Autodesk Inventor part; units mm, degrees
ref_plane "YZ Plane" through (0, 0, 0) normal (1, 0, 0) x (0, 1, 0)
ref_plane "XZ Plane" through (0, 0, 0) normal (0, 1, 0) x (-1, 0, 0)
ref_plane "XY Plane" through (0, 0, 0) normal (0, 0, 1) x (1, 0, 0)
sketch "Sketch1" plane through (0, 0, 0) normal (0, 1, 0) x (-1, 0, 0)
  line L0 (0, 0) -> (-19.6, 0)
  line L1 (-19.6, 0) -> (-19.6, -4)
  line L2 (-19.6, -4) -> (0, -4)
  line L3 (0, -4) -> (0, 0)
  dimension "d0" = 4
  dimension "d1" = 19.6
extrude "Extrusion1" add sketch "Sketch1" along normal blind 34
sketch "Sketch2" plane through (0, 0, -4) normal (-1, 0, 0) x (0, 0, 1)
  line L0 (4, 34) -> (0, 34)
  line L1 (0, 34) -> (8, 34)
  line L2 (8, 34) -> (8, 42)
  line L3 (8, 42) -> (0, 42)
  line L4 (0, 42) -> (0, 34)
  line L5 (4, 0) -> (4, 34)
  dimension "d4" = 4
  dimension "d5" = 8
  dimension "d6" = 8
extrude "Extrusion2" add sketch "Sketch2" against normal blind 32
sketch "Sketch3" plane through (32, 0, -4) normal (1, 0, 0) x (0, 0, -1)
  circle A0 centre (-4, 38) radius 2.5
  line L0 (0, 42) -> (-8, 42)
  line L1 (-8, 42) -> (-8, 34)
  line L2 (0, 34) -> (0, 42)
  line L3 (-8, 34) -> (0, 34)
  point P0 (-4, 0)
  dimension "d9" = 4
  dimension "d10" = 4
  dimension "d11" = 4
  dimension "d12" = 4
  dimension "d13" = 5
extrude "Extrusion3" cut sketch "Sketch3" against normal blind 30.8 contours A0
sketch "Sketch4" plane through (0, 0, 0) normal (0, -1, 0) x (1, 0, 0)
  line L0 (18.4, -3.2) -> (15.6, -3.2)
  line L1 (15.6, -3.2) -> (15.6, -1.6)
  line L2 (15.6, -1.6) -> (18.4, -1.6)
  line L3 (18.4, -1.6) -> (18.4, -3.2)
  line L4 (11.2, -3.2) -> (8.4, -3.2)
  line L5 (8.4, -3.2) -> (8.4, -1.6)
  line L6 (8.4, -1.6) -> (11.2, -1.6)
  line L7 (11.2, -1.6) -> (11.2, -3.2)
  line L8 (4, -3.2) -> (1.2, -3.2)
  line L9 (1.2, -3.2) -> (1.2, -1.6)
  line L10 (1.2, -1.6) -> (4, -1.6)
  line L11 (4, -1.6) -> (4, -3.2)
  line L12 (19.6, 0) -> (19.6, -4)
  line L13 (19.6, -4) -> (0, -4)
  line L14 (0, 0) -> (19.6, 0)
  line L15 (0, -4) -> (0, 0)
  dimension "d16" = 2.8
  dimension "d17" = 1.2
  dimension "d18" = 0.8
  dimension "d19" = 1.6
  dimension "d20" = 1.6
  dimension "d21" = 2.8
  dimension "d22" = 2.8
  dimension "d23" = 4.4
  dimension "d24" = 1.2
  dimension "d25" = 4.4
extrude "Extrusion4" cut sketch "Sketch4" against normal blind 38 contours L0 L1 L2 L3 | L4 L5 L6 L7 | L8 L9 L10 L11
sketch "Sketch5" plane through (19.6, 0, -4) normal (0, 0, -1) x (-1, 0, 0)
  line L0 (1.2, 0) -> (1.2, 38)
  line L1 (4, 0) -> (4, 38)
  line L2 (1.2, 27) -> (4, 27)
  line L3 (4, 27) -> (4, 7)
  line L4 (4, 7) -> (1.2, 7)
  line L5 (1.2, 7) -> (1.2, 27)
  line L6 (8.4, 0) -> (8.4, 36.0791)
  line L7 (11.2, 0) -> (11.2, 38)
  line L8 (8.4, 27) -> (11.2, 27)
  line L9 (11.2, 27) -> (11.2, 7)
  line L10 (11.2, 7) -> (8.4, 7)
  line L11 (8.4, 7) -> (8.4, 27)
  line L12 (15.6, 0) -> (15.6, 36.0791)
  line L13 (15.6, 27) -> (18.4, 27)
  line L14 (18.4, 27) -> (18.4, 7)
  line L15 (18.4, 7) -> (15.6, 7)
  line L16 (15.6, 7) -> (15.6, 27)
  line L17 (0, 0) -> (19.6, 0)
  line L18 (0, 34) -> (-12.4, 34)
  line L19 (19.6, 0) -> (19.6, 42)
  point P0 (18.4, 0)
  point P1 (15.6, 7)
  point P2 (8.4, 7)
  point P3 (1.2, 7)
  point P4 (4, 27)
  dimension "d28" = 7
  dimension "d29" = 20
  dimension "d30" = 7
  dimension "d49" = 1.2
extrude "Extrusion5" cut sketch "Sketch5" against normal blind 0.8 contours L12 L13 L14 L15 | L0 L2 L1 L4 | L6 L8 L7 L10
sketch "Sketch6" plane through (19.6, 0, -4) normal (0, 0, -1) x (-1, 0, 0)
  line L0 (5.2, 27) -> (7.2, 27)
  line L1 (7.2, 27) -> (7.2, 7)
  line L2 (7.2, 7) -> (5.2, 7)
  line L3 (5.2, 7) -> (5.2, 27)
  line L4 (12.4, 27) -> (14.4, 27)
  line L5 (14.4, 27) -> (14.4, 7)
  line L6 (14.4, 7) -> (12.4, 7)
  line L7 (12.4, 7) -> (12.4, 27)
  line L8 (4, 27) -> (4, 7)
  line L9 (8.4, 7) -> (8.4, 27)
  line L10 (11.2, 27) -> (11.2, 7)
  line L11 (15.6, 7) -> (15.6, 27)
  line L12 (19.6, 0) -> (19.6, 42)
  line L13 (0, 0) -> (0, 34)
  dimension "d33" = 1.2
  dimension "d34" = 1.2
  dimension "d35" = 1.2
  dimension "d36" = 1.2
  dimension "d37" = 2
  dimension "d38" = 2
  dimension "d39" = 19.6
extrude "Extrusion6" cut sketch "Sketch6" against normal up to surface (4 mm away)
sketch "Sketch7" plane through (0, 0, 0) normal (0, -1, 0) x (1, 0, 0)
  line L0 (19.6, -4) -> (32, -4)
  line L1 (0, 0) -> (19.6, 0)
  line L2 (19.6, -4) -> (0, -4)
  line L3 (0, -4) -> (0, 0)
  line L4 (0, 0) -> (19.6, 0)
  line L5 (19.6, 0) -> (19.6, -4)
extrude "Extrusion7" add sketch "Sketch7" against normal blind 7
properties part number "20210811_H2_gasmanifold_old_v1"
The listing builds one solid part. Answer for the finished solid, in the listing's coordinates (mm). A direction names the side the tool comes from. Give positions to 0.01 mm unless a question says otherwise; leave off trailing zeros. Order: outer loops, then holes, each group sorted by start corner. A loop starts at its lowest first (then second) coordinate and runs counter-clockwise, first axis right, second up. Notation, with made-up numbers: (24.5, -23) -> (33.5, -23) arc R21 cw to (33.5, -15) -> close; hole circle Ø5 at (62, 77). An arc over 180 degrees is marked (long way). Put each result on its own line as item: value.
Item 1: A cutting plane is placed at C-C on z = 1.5. Give the vertices of the cut face in (x, y), plus the area to 3 significant figures.
Established:
outline: (0, 34) -> (32, 34) -> (32, 36) -> (1.2, 36) -> (1.2, 40) -> (32, 40) -> (32, 42) -> (0, 42) -> close
area: 133 mm^2
Item 2: A cutting plane is placed at D-D on x = 3.5. Give the vertices of the cut face in (y, z).
Established:
outline: (0, -4) -> (7, -4) -> (7, -1.6) -> (36.08, -1.6) arc R2.5 cw (long way) to (38, -2.5) -> (38, -3.2) -> (27, -3.2) -> (27, -4) -> (42, -4) -> (42, 4) -> (34, 4) -> (34, 0) -> (0, 0) -> close
Item 3: Straight lines are drawn through the part: line 1 (X direction, y = 24.5, z = -3.25); line 2 (X direction, y = 9.5, z = -0.75); line 3 (Z direction, x = 15, y = 38). For each, find the intervals that lie inside material, in ascending order.
Established:
line 1: x = 0 to 1.2, 4 to 5.2, 7.2 to 8.4, 11.2 to 12.4, 14.4 to 15.6, 18.4 to 19.6
line 2: x = 0 to 5.2, 7.2 to 12.4, 14.4 to 19.6
line 3: z = -4 to -2.5, 2.5 to 4
Item 4: A cutting plane is placed at B-B on x = 21. Give the vertices of the cut face in (y, z), plus the area to 3 significant figures.
Established:
outline: (34, -4) -> (42, -4) -> (42, 4) -> (34, 4) -> close; hole circle Ø5 at (38, 0)
area: 44.4 mm^2
Item 5: A cutting plane is placed at A-A on y = 33.5. Give the vertices of the cut face in (x, z).
Established:
outline: (0, -4) -> (19.6, -4) -> (19.6, 0) -> (0, 0) -> close; hole (1.2, -3.2) -> (4, -3.2) -> (4, -1.6) -> (1.2, -1.6) -> close; hole (8.4, -3.2) -> (11.2, -3.2) -> (11.2, -1.6) -> (8.4, -1.6) -> close; hole (15.6, -3.2) -> (18.4, -3.2) -> (18.4, -1.6) -> (15.6, -1.6) -> close
Item 6: Given P1, Ø2, axis at y = 12.5, z = -2.5, coming from the +X side; P2, Ø1, axis at x = 10.5, y = 11, coming from the +Z side; P3, Ø0.8, axis at x = 10, y = 17, coming from the -Z side, each flat-ended and moving along its own axis, determine where each tip first touches the part or whether it passes through.
Established:
P1: stops at x = 19.6
P2: stops at z = 0
P3: stops at z = -1.6
Item 7: For a pull along Z with two mould halves and no side action, classify faces 1 (the face through (18.4, 22, -3)), 2 (the face through (10, 21, -1.6)), 3 (the face through (13, 30, -4)), 4 (the face through (10, 0, -2)) as released by +Z, released by -Z, zero draft, split by the parting line, or undercut.
Established:
face 1: undercut
face 2: undercut
face 3: released by -Z
face 4: zero draft
Item 8: For faces 5 (the face through (3, 7, -3)), 6 (the face through (16.8, 38.1, 2.5)), 7 (the face through (32, 40, -2)), 8 (the face through (6, 7, -2)), 9 (the face through (11.2, 22, -3)), determine the directions among +Z, -Z, +X, -X, +Y, -Y from which every point of the face is accessible in a straight line to the end or side of a thin tool.
Established:
face 5: -Z
face 6: +X
face 7: +Z, -Z, +X, +Y, -Y
face 8: +Z, -Z
face 9: none
